from build123d import *

# Parameters (mm, degrees)
BASE_FLANGE1_DEPTH      = 19
CUT_EXTRUDE1_DEPTH      = 47.270941205
CUT_EXTRUDE1_DEPTH_BACK = 47.270941205
SKETCH5_W               = 32
SKETCH5_H               = 11
SKETCH6_R               = 2
CUT_EXTRUDE2_DEPTH      = 47.270941205
CUT_EXTRUDE4_DEPTH      = 47.270941205
CUT_EXTRUDE4_DEPTH_BACK = 47.270941205
SKETCH7_W               = 30.575
SKETCH7_H               = 8
SKETCH8_W               = 30.575
SKETCH8_H               = 8
TAB1_DEPTH              = 2


# Sheet-metal steps are written as plain solids
with BuildPart() as part:
    # Sketch2 → Base-Flange1 (new body)
    with BuildSketch(Plane(origin=(0, 0, 0), x_dir=(1, 0, 0), z_dir=(0, 1, 0))):
        with BuildLine():
            Line((0, 0), (12.85, 0))
            ThreePointArc((12.85, 0), (14.37027958, -0.62972042), (15, -2.15))
            Line((15, -2.15), (15, -3.85))
            ThreePointArc((15, -3.85), (15.043933983, -3.956066017), (15.15, -4))
            Line((15.15, -4), (42, -4))
            Line((42, -4), (42, -6))
            Line((42, -6), (15.15, -6))
            ThreePointArc((15.15, -6), (13.62972042, -5.37027958), (13, -3.85))
            Line((13, -3.85), (13, -2.15))
            ThreePointArc((13, -2.15), (12.956066017, -2.043933983), (12.85, -2))
            Line((12.85, -2), (0, -2))
            Line((0, -2), (0, 0))
        make_face()
    extrude(amount=BASE_FLANGE1_DEPTH)

    # Sketch5 → Cut-Extrude1 (cut, two sides: drawn at the far end of the back side and taken through both)
    with BuildSketch(Plane.XY.offset(2).offset(-CUT_EXTRUDE1_DEPTH_BACK)):
        with Locations((26, 5.5)):
            Rectangle(SKETCH5_W, SKETCH5_H)
    extrude(amount=CUT_EXTRUDE1_DEPTH + CUT_EXTRUDE1_DEPTH_BACK, mode=Mode.SUBTRACT)

    # Sketch6 → Cut-Extrude2 (cut, through all)
    with BuildSketch(Plane.XY.offset(2)):
        with Locations((5, 5)):
            Circle(SKETCH6_R)
    extrude(amount=-CUT_EXTRUDE2_DEPTH, mode=Mode.SUBTRACT)

    # Sketch7 → Cut-Extrude4 (cut, two sides: drawn at the far end of the back side and taken through both)
    with BuildSketch(Plane.XY.offset(2).offset(-CUT_EXTRUDE4_DEPTH_BACK)):
        with Locations((26.7125, 15)):
            Rectangle(SKETCH7_W, SKETCH7_H)
    extrude(amount=CUT_EXTRUDE4_DEPTH + CUT_EXTRUDE4_DEPTH_BACK, mode=Mode.SUBTRACT)

    # Sketch8 → Tab1 (add)
    with BuildSketch(Plane.XY.offset(2)):
        with Locations((26.7125, 15)):
            Rectangle(SKETCH8_W, SKETCH8_H)
    extrude(amount=-TAB1_DEPTH)


solid = part.part
Source: CAD feature listing. Evaluate the final solid. Frame: model axes, mm. A direction names the side the tool comes from. Round coordinates to 2 decimals unless told otherwise and drop trailing zeros. Loops run counter-clockwise (first coordinate to the right, second up) from the corner with the lowest first, then second, coordinate; pieces in that order, holes last. Notation, with made-up numbers: M 87,83.25 L 145,83.25 A23 ccw 145,106.25 Z; hole C 88,29.25 d1. An arc over 180 degrees is marked long. Answer as CSV lines item,"result".
Q1. Cut plane D-D (y = 2.5). Return the cut outline in (x, z).
Verdict:
outline,"M 0,0 L 10,0 L 10,2 L 0,2 Z"
Q2. Line query: line 1 along Y through (x, z) = (5, 0.65); line 2 along Y through (x, z) = (39.5, 0.95); line 3 along X through (y, z) = (10.5, 1.45). Output: solid intervals per line, ascending.
Verdict:
line 1,"y = 0 to 3, 7 to 19"
line 2,"y = 11 to 19"
line 3,"x = 0 to 10"
Q3. Cut plane C-C (z = 0.8). Return the cut outline in (x, y).
Verdict:
outline,"M 0,0 L 10,0 L 10,11 L 42,11 L 42,19 L 0,19 Z; hole C 5,5 d4"
Q4. Reachability of faces 5 (the face through (16, 14, 2)), 6 (the face through (26, 11, 1)) from +Z, -Z, +X, -X, +Y, -Y: full face, straight path, thin tool, end or side. Return the list, or none.
Verdict:
face 5,"+Z, +X, -X, +Y, -Y"
face 6,"+Z, -Z, +X, -Y"
Q5. Cut plane B-B (y = 5). Return the cut outline in (x, z), plus the area to 3 significant figures.
Verdict:
outline,"M 0,0 L 3,0 L 3,2 L 0,2 Z; M 7,0 L 10,0 L 10,2 L 7,2 Z"
area,"12.0 mm^2"
Q6. Pull-direction query (X, two-part tool) for faces 1 (the face through (0, 9, 1)), 2 (the face through (3, 5, 1)), 3 (the face through (21, 19, 1)), 4 (the face through (42, 15, 1)); classes: +X half, -X half, draft (parallel to the pull), parting line (faces both ways), or undercut.
Verdict:
face 1,"-X half"
face 2,"undercut"
face 3,"draft"
face 4,"+X half"
Q7. Contact query for flat-ended pins moving along their axis: pin 1 (3 mm diameter, centred on x = 7, y = 5.5, fed in from -Z); pin 2 (0.6 mm diameter, centred on x = 33.5, z = 0.5, fed in from -Y). Output: stop coordinate, or through.
Verdict:
pin 1,"stops at z = 0"
pin 2,"stops at y = 11"
Q8. Cut plane A-A (x = 5). Return the cut outline in (y, z), plus the area to 3 significant figures.
Verdict:
outline,"M 0,0 L 3,0 L 3,2 L 0,2 Z; M 7,0 L 19,0 L 19,2 L 7,2 Z"
area,"30.0 mm^2"
